from build123d import *

# Parameters (mm, degrees)
F1_DEPTH = 31.75
F1_TAPER = 0.5
F2_DEPTH = 36.5125
F3_DEPTH = 3.175
F5_DEPTH = 15.876
F7_R     = 6.35
F8_DEPTH = 3.175


with BuildPart() as f1:
    # F0 (on Top) → F1 (new body)
    with BuildSketch(Plane.XY):
        with BuildLine():
            Line((0, -13.3223), (0, 13.3223))
            ThreePointArc((0, 13.3223), (-13.3223, 0), (0, -13.3223))
        make_face()
        with BuildLine():
            ThreePointArc((0, -13.3223), (9.420288671, -9.420288671), (13.3223, 0))
            ThreePointArc((13.3223, 0), (9.420288671, 9.420288671), (0, 13.3223))
            Line((0, 13.3223), (0, -13.3223))
        make_face()
    extrude(amount=F1_DEPTH, taper=F1_TAPER)

    # F0 (on Top) → F2 (join)
    with BuildSketch(Plane.XY):
        with BuildLine():
            ThreePointArc((0, -13.3223), (9.420288671, -9.420288671), (13.3223, 0))
            ThreePointArc((13.3223, 0), (9.420288671, 9.420288671), (0, 13.3223))
            Line((0, 13.3223), (0, -13.3223))
        make_face()
        with BuildLine():
            ThreePointArc((0, 13.3223), (9.420288671, 9.420288671), (13.3223, 0))
            ThreePointArc((13.3223, 0), (9.420288671, -9.420288671), (0, -13.3223))
            Line((0, -13.3223), (0, -15.875))
            ThreePointArc((0, -15.875), (11.2253201513, -11.2253201513), (15.875, 0))
            ThreePointArc((15.875, 0), (11.2253201513, 11.2253201513), (0, 15.875))
            Line((0, 15.875), (0, 13.3223))
        make_face()
    extrude(amount=-F2_DEPTH)

    # F0 (on Top) → F3 (join)
    with BuildSketch(Plane.XY):
        with BuildLine():
            ThreePointArc((0, -13.3223), (-13.3223, 0), (0, 13.3223))
            Line((0, 13.3223), (0, 15.875))
            ThreePointArc((0, 15.875), (-15.875, 0), (0, -15.875))
            Line((0, -15.875), (0, -13.3223))
        make_face()
        with BuildLine():
            Line((0, -13.3223), (0, 13.3223))
            ThreePointArc((0, 13.3223), (-13.3223, 0), (0, -13.3223))
        make_face()
    extrude(amount=-F3_DEPTH)

    # F4 (on face) → F5 (cut, through all)
    with BuildSketch(Plane(origin=(0, 0, 0), x_dir=(0, -1, 0), z_dir=(-1, 0, 0))):
        with BuildLine():
            ThreePointArc((-3.175, -20.6375), (0, -23.8125), (3.175, -20.6375))
            Line((3.175, -20.6375), (-3.175, -20.6375))
        make_face()
        with BuildLine():
            Line((-3.175, -20.6375), (3.175, -20.6375))
            ThreePointArc((3.175, -20.6375), (0, -17.4625), (-3.175, -20.6375))
        make_face()
        with BuildLine():
            ThreePointArc((5.44e-08, -36.5125), (-11.2253201321, -31.8628201706), (-15.875, -20.6375))
            Line((-15.875, -20.6375), (-15.875, -36.5125))
            Line((-15.875, -36.5125), (5.44e-08, -36.5125))
        make_face()
        with BuildLine():
            Line((15.875, -36.5125), (15.875, -20.6375))
            ThreePointArc((15.875, -20.6375), (11.2253201706, -31.8628201321), (5.44e-08, -36.5125))
            Line((5.44e-08, -36.5125), (15.875, -36.5125))
        make_face()
    extrude(amount=-F5_DEPTH, mode=Mode.SUBTRACT)

    # F7 (on offset) → F8 (cut)
    with BuildSketch(Plane.YZ.offset(15.875)):
        with Locations((0, -20.6375)):
            Circle(F7_R)
    extrude(amount=-F8_DEPTH, mode=Mode.SUBTRACT)


solid = f1.part
For this review, take the finished solid that the model builds, in its own axes (mm). A direction names the side the tool comes from. Give positions to 0.01 mm unless a question says otherwise; leave off trailing zeros. Loops run counter-clockwise (first coordinate to the right, second up) from the corner with the lowest first, then second, coordinate; pieces in that order, holes last.
Item 1: Take a section at B-B, the plane z = 22. State the section outline as (x, y) points.
Item 2: Tool access review of faces 1 (the flat face through (0, 0, 31.75)), 2 (the cylindrical face through (6.261, 0.688, -23.737)), 3 (the flat face through (-4, 13, 0)), 4 (the flat face through (12.7, -3, -19)), 5 (the flat face through (-6, 0, -3.175)): name each direction out of +Z, -Z, +X, -X, +Y, -Y from which nothing blocks a thin tool from reaching the whole face with its end or side.
Item 3: Insertion check: pin 1 (3 mm diameter, centred on x = 4.5, z = 21, fed in from +Y); pin 2 (12 mm diameter, centred on y = -3, z = 12.5, fed in from -X); pin 3 (1.5 mm diameter, centred on x = 2, z = -5.5, fed in from +Y). Each pin has a flat end and moves straight along its axis. Give the tip position at first contact, or say it passes through.
Item 4: Take a section at A-A, the plane z = -6. State the section outline as (x, y) points (3 decimals), and give its area (3 significant figures).
Item 5: For line 1 along Z through (x, y) = (2, 0); line 2 along Z through (x, y) = (13.4, 0); line 3 along X through (y, z) = (-9.5, -5.5), list the stretches that pass through material, from the lowest coordinate up.
Calculated:
1. outline: circle Ø26.26 at (0, 0)
2. face 1: +Z, +X, -X, +Y, -Y
2. face 2: +X, -X
2. face 3: +Z
2. face 4: +X
2. face 5: -Z, -X, +Y, -Y
3. pin 1: stops at y = 12.79
3. pin 2: stops at x = -13.26
3. pin 3: stops at y = 15.83
4. outline: (0, -15.875) arc R15.875 ccw to (0, 15.875) - close
4. area: 396 mm2
5. line 1: z = -36.51 to -23.81, -17.46 to 31.75
5. line 2: z = -36.51 to -26.99, -14.29 to 0
5. line 3: x = 0 to 12.72
